Design review of the part built by this model. Coordinates are the model's own, in mm. A direction names the side the tool comes from. Give positions to 0.01 mm unless a question says otherwise; leave off trailing zeros. Loops run counter-clockwise (first coordinate to the right, second up) from the corner with the lowest first, then second, coordinate; pieces in that order, holes last. Notation, with made-up numbers: M -5,45 L 41,45 A16 ccw 41,50 Z; hole C -15,76 d4. An arc over 180 degrees is marked long. Use one line per item in the form item = value. Start each with the question number.
from build123d import *

# Parameters (mm, degrees)
SKETCH1_R            = 2.5
BOSS_EXTRUDE1_DEPTH  = 6.35
M3_CLEARANCE_HOLE1_D = 3.4
CIRPATTERN1_COUNT    = 4
M3_CLEARANCE_HOLE3_D = 3.4
FILLET1_R            = 3


with BuildPart() as part:
    # Sketch1 → Boss-Extrude1 (new body)
    with BuildSketch(Plane(origin=(0, 0, 0), x_dir=(1, 0, 0), z_dir=(0, 1, 0))):
        with BuildLine():
            Line((-38.1, 67.7), (38.1, 67.7))
            Line((38.1, 67.7), (38.1, -38.1))
            Line((38.1, -38.1), (-38.1, -38.1))
            Line((-38.1, -38.1), (-38.1, -2.5))
            Line((-38.1, -2.5), (-14.790199458, -2.5))
            ThreePointArc((-14.790199458, -2.5), (15, 0), (-14.790199458, 2.5))
            Line((-14.790199458, 2.5), (-38.1, 2.5))
            Line((-38.1, 2.5), (-38.1, 67.7))
        make_face()
        with Locations(Location((33.1, 62.7, 0), (0, 0, 270))):
            Circle(SKETCH1_R, mode=Mode.SUBTRACT)
        with BuildLine():
            ThreePointArc((26.105667768, 47.700606125), (21.397382771, 50.997382771), (18.100606125, 55.705667768))
            ThreePointArc((18.100606125, 55.705667768), (14.778291003, 56.914891581), (13.569067189, 53.592576459))
            ThreePointArc((13.569067189, 53.592576459), (17.861848865, 47.461848865), (23.992576459, 43.169067189))
            ThreePointArc((23.992576459, 43.169067189), (27.314891581, 44.378291003), (26.105667768, 47.700606125))
        make_face(mode=Mode.SUBTRACT)
    extrude(amount=BOSS_EXTRUDE1_DEPTH)

    # M3 Clearance Hole1 (through all)
    with Locations(Plane(origin=(0, 6.35, 0), x_dir=(1, 0, 0), z_dir=(0, 1, 0))):
        with Locations((13.470384182, 13.470384182)):
            m3_clearance_hole1 = Hole(M3_CLEARANCE_HOLE1_D / 2)

    # CirPattern1: M3 Clearance Hole1 ×4 about axis
    cirpattern1_axis = Axis((0, 0, 0), (0, 1, 0))
    for i in range(1, CIRPATTERN1_COUNT):
        add(m3_clearance_hole1.rotate(cirpattern1_axis, i * 360 / CIRPATTERN1_COUNT), mode=Mode.SUBTRACT)

    # M3 Clearance Hole3 (through all)
    with Locations(Plane(origin=(0, 6.35, 0), x_dir=(1, 0, 0), z_dir=(0, 1, 0))):
        with Locations((11, 34.1), (-11, -34.1), (11, -34.1), (-11, 34.1)):
            Hole(M3_CLEARANCE_HOLE3_D / 2)

    # Fillet1
    fillet1_edges = [part.edges().sort_by_distance(p)[0] for p in [
        (-14.790199458, 3.175, -2.5),
        (-38.1, 3.175, -2.5),
        (-38.1, 3.175, 2.5),
        (-14.790199458, 3.175, 2.5),
    ]]
    fillet(fillet1_edges, radius=FILLET1_R)


solid = part.part
Q1. For faces 1 (the cylindrical face through (-37.24, 3.22, -3.4)), 2 (the cylindrical face through (-15.393, 3.219, -3.061)), 3 (the flat face through (1, 6.35, -16)), list the 3-axis set-ups (+Z, -Z, +X, -X, +Y, -Y) from which the entire face can be reached by the end or side of a thin tool; tool diameter is ignored.
Q2. Take a section at B-B on z = -34.1. Give the boundary of the cut face in (x, y).
Q3. Take a section at C-C on x = -27.5. Give the boundary of the cut face in (y, z), plus the area to 3 significant figures.
Q4. Wall thickness on probe 1 along X at (y, z) = (3.5, -34.1); probe 2 along Z at (x, y) = (10, 5.5); probe 3 along Z at (x, y) = (11, 4): over which ranges is each line inside the solid? List them lowest first.
Q5. The part is to be moulded in two halves that separate along Z. For faces 4 (the cylindrical face through (17.788, 3.131, -47.536)), 5 (the flat face through (38.1, 3, -16)), say which applies: pulls with the +Z half, pulls with the -Z half, needs draft (parallel to the pull), parting line crosses it, or undercut.
Q6. Take a section at D-D on y = 4.5. State how many separate pieces and enclosed holes the cut face has, plus the area to 3 significant figures.
Q7. Take a section at A-A on z = -62.7. Give the boundary of the cut face in (x, y), plus the area to 3 significant figures.
Response values:
q1.face_1 = -X, +Y, -Y
q1.face_2 = +Y, -Y
q1.face_3 = +Z, -Z, +X, -X, +Y
q2.outline = M -38.1,0 L -12.7,0 L -12.7,6.35 L -38.1,6.35 Z; M -9.3,0 L 9.3,0 L 9.3,6.35 L -9.3,6.35 Z; M 12.7,0 L 38.1,0 L 38.1,6.35 L 12.7,6.35 Z
q3.outline = M 0,-67.7 L 6.35,-67.7 L 6.35,-2.5 L 0,-2.5 Z; M 0,2.5 L 6.35,2.5 L 6.35,38.1 L 0,38.1 Z
q3.area = 640 mm^2
q4.probe_1 = -38.1 to -12.7, -9.3 to 9.3, 12.7 to 38.1
q4.probe_2 = -67.7 to -35.47, -32.73 to -11.18, 11.18 to 32.73, 35.47 to 38.1
q4.probe_3 = -67.7 to -35.8, -32.4 to -10.2, 10.2 to 32.4, 35.8 to 38.1
q5.face_4 = undercut
q5.face_5 = needs draft
q6.separate_pieces = 1
q6.enclosed_holes = 10
q6.area = 7,050 mm^2
q7.outline = M -38.1,0 L 30.6,0 L 30.6,6.35 L -38.1,6.35 Z; M 35.6,0 L 38.1,0 L 38.1,6.35 L 35.6,6.35 Z
q7.area = 452 mm^2
